Geometry check sheet. Reference: the model listing, model coordinates, mm. Face numbers are marked on the shaded views. Give positions to 0.01 mm unless a question says otherwise; leave off trailing zeros. Loops run counter-clockwise (first coordinate to the right, second up) from the corner with the lowest first, then second, coordinate; pieces in that order, holes last.
1. Go/stop test with flat-tipped pins: pin 1 Ø4 at (x, z) = (0, -23.81) entering from +Y; pin 2 Ø3 at (x, y) = (0, -4.76) entering from +Z; pin 3 Ø2 at (x, y) = (-18, -2) entering from -Z; pin 4 Ø5 at (x, y) = (-8, -5) entering from -Z. Record where each tip stops, or that it passes through.
2. Cross-section at C-C, the plane y = -7.75. Record the cut outline in (x, z), plus the area to 3 significant figures.
3. Release check for a two-part mould opening along Z. For the marked faces 1, 2 and 3 record: +Z half, -Z half, draft (parallel to the pull), parting line (faces both ways), or undercut.
4. Cross-section at A-A, the plane x = 0. Record the cut outline in (y, z) (1 decimal), plus the area to 3 significant figures.
5. Material ranges on L1, parallel to Y at x = 0, z = 14 (1 decimal); L2, parallel to Y at x = 0.5, z = 10 (3 decimals); L3, parallel to Z at x = -3, y = -7.75, recorded low to high.
6. Cross-section at B-B, the plane z = -22. Record the cut outline in (x, y) (3 decimals).
from build123d import *

# Parameters (mm, degrees)
SKETCH1_R                        = 4.191
BOSS_EXTRUDE1_DEPTH              = 9.525
F_10_CLEARANCE_HOLE1_D           = 4.9784
TAP_DRILL_FOR_M4X0_7_TAP1_REACH  = 62.679
TAP_DRILL_FOR_M4X0_7_TAP1_BORE_R = 1.65
CHAMFER1_SIZE                    = 6.35
CHAMFER1_EDGE_2_SIZE             = 6.35
CHAMFER1_EDGE_3_SIZE             = 6.35
FILLET2_R                        = 0.79375


with BuildPart() as part:
    # Sketch1 → Boss-Extrude1 (new body)
    with BuildSketch(Plane(origin=(0, 0, 0), x_dir=(1, 0, 0), z_dir=(0, 1, 0))):
        Polygon((0, 34.925), (30.245937227, -17.4625), (-30.245937227, -17.4625), align=None)
        with Locations(Location((0, 0, 0), (0, 0, 270))):
            Circle(SKETCH1_R, mode=Mode.SUBTRACT)
    extrude(amount=-BOSS_EXTRUDE1_DEPTH)

    # #10 Clearance Hole1 (through all)
    with Locations(Plane(origin=(0, 0, -23.8125), x_dir=(0, 0, 1), z_dir=(0, 1, 0))):
        with Locations((0, 0), (35.71875, 20.622229928), (35.71875, -20.622229928)):
            Hole(F_10_CLEARANCE_HOLE1_D / 2)

    # Tap Drill for M4x0.7 Tap1 bore (on position points) → Tap Drill for M4x0.7 Tap1 (cut, up to next)
    with BuildSketch(Plane(origin=(0, -4.7625, 17.4625), x_dir=(1, 0, 0), z_dir=(0, 0, 1)), mode=Mode.PRIVATE) as tap_drill_for_m4x0_7_tap1_sk1:
        Circle(TAP_DRILL_FOR_M4X0_7_TAP1_BORE_R)
    tap_drill_for_m4x0_7_tap1_tool1 = extrude(tap_drill_for_m4x0_7_tap1_sk1.sketch, amount=-TAP_DRILL_FOR_M4X0_7_TAP1_REACH, mode=Mode.PRIVATE) & part.part
    add(tap_drill_for_m4x0_7_tap1_tool1.solids().sort_by_distance((0, -4.7625, 17.4625))[0], mode=Mode.SUBTRACT)

    # Chamfer1
    chamfer1_edges = [part.edges().sort_by_distance(p)[0] for p in [
        (0, -4.7625, -34.925),
    ]]
    chamfer(chamfer1_edges, length=CHAMFER1_SIZE)

    # Chamfer1 edge 2
    chamfer1_edge_2_edges = [part.edges().sort_by_distance(p)[0] for p in [
        (30.245937227, -4.7625, 17.4625),
    ]]
    chamfer(chamfer1_edge_2_edges, length=CHAMFER1_EDGE_2_SIZE)

    # Chamfer1 edge 3
    chamfer1_edge_3_edges = [part.edges().sort_by_distance(p)[0] for p in [
        (-30.245937227, -4.7625, 17.4625),
    ]]
    chamfer(chamfer1_edge_3_edges, length=CHAMFER1_EDGE_3_SIZE)

    # Fillet2
    fillet2_edges = [part.edges().sort_by_distance(p)[0] for p in [
        (-3.175, -4.7625, -29.425738686),
        (-27.070937227, -4.7625, 11.963238686),
        (23.895937227, -4.7625, 17.4625),
        (-23.895937227, -4.7625, 17.4625),
        (3.175, -4.7625, -29.425738686),
        (27.070937227, -4.7625, 11.963238686),
    ]]
    fillet(fillet2_edges, radius=FILLET2_R)


solid = part.part
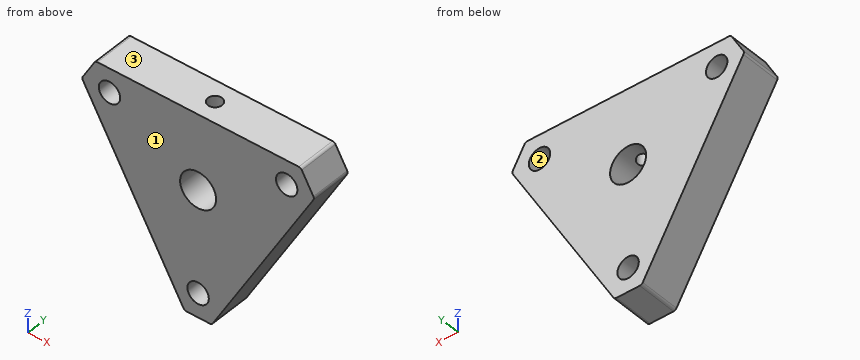
Result:
1. pin 1: passes through
1. pin 2: stops at z = -3.91
1. pin 3: stops at z = -5.48
1. pin 4: stops at z = -25.4
2. outline: (-26.84, 11.57) - (-3.4, -29.03) arc R0.79 ccw to (-2.72, -29.43) - (2.72, -29.43) arc R0.79 ccw to (3.4, -29.03) - (26.84, 11.57) arc R0.79 ccw to (26.84, 12.36) - (24.13, 17.07) arc R0.79 ccw to (23.44, 17.46) - (-23.44, 17.46) arc R0.79 ccw to (-24.13, 17.07) - (-26.84, 12.36) arc R0.79 ccw to start; hole circle Ø4.98 at (-20.62, 11.91); hole circle Ø8.38 at (0, 0); hole circle Ø4.98 at (0, -23.81); hole circle Ø4.98 at (20.62, 11.91)
2. area: 1,420 mm2
3. face 1: draft
3. face 2: undercut
3. face 3: +Z half
4. outline: (-9.5, -29.4) - (0, -29.4) - (0, -26.3) - (-9.5, -26.3) - close; (-9.5, -21.3) - (0, -21.3) - (0, -4.2) - (-9.5, -4.2) - close; (-9.5, 4.2) - (-6.4, 4.2) - (-6.4, 17.5) - (-9.5, 17.5) - close; (-3.1, 4.2) - (0, 4.2) - (0, 17.5) - (-3.1, 17.5) - close
4. area: 276 mm2
5. L1: y = -9.5 to -6.4, -3.1 to 0
5. L2: y = -9.525 to -6.335, -3.19 to 0
5. L3: z = -29.37 to -2.93, 2.93 to 17.46
6. outline: (-7.462, -9.525) - (-1.706, -9.525) - (-1.706, 0) - (-7.462, 0) - close; (1.706, -9.525) - (7.462, -9.525) - (7.462, 0) - (1.706, 0) - close
